Answer from the drawing. Dimensions are ordinates in mm from the lowest x, y and z of the part. Coordinates: 2 decimals unless noted, no trailing zeros. Write each loop counter-clockwise with the first axis right and the second up, starting at its lowest first coordinate (ties: lowest second). Pieces come first, ordered by that corner, then holes.
(1) For a pull along Y with two mould halves and no side action, classify the marked faces 1, 2 and 3 as +Y half, -Y half, draft (parallel to the pull), parting line (faces both ways), or undercut.
(2) Straight lines are drawn through the part: line 1 (X direction, y = 3, z = 36); line 2 (Y direction, x = 19, z = 32); line 3 (Y direction, x = 4, z = 6). For each, find the intervals that lie inside material, in ascending order.
(3) The part is cut by section C-C on z = 3.81. Give the number of separate pieces and of enclosed holes in the cut face, plus the area to 3 significant figures.
(4) The part is cut by section A-A on x = 19.05. Determine the outline of the cut face in (y, z), plus the area to 3 significant figures.
(5) Given P1, Ø4, axis at x = 28.575, z = 3.81, coming from the -Y side; P2, Ø4, axis at x = 9.525, z = 30.48, coming from the +Y side; P3, Ø7.5, axis at x = 19.05, y = 19.05, coming from the +Z side, each flat-ended and moving along its own axis, determine where each tip first touches the part or whether it passes through.
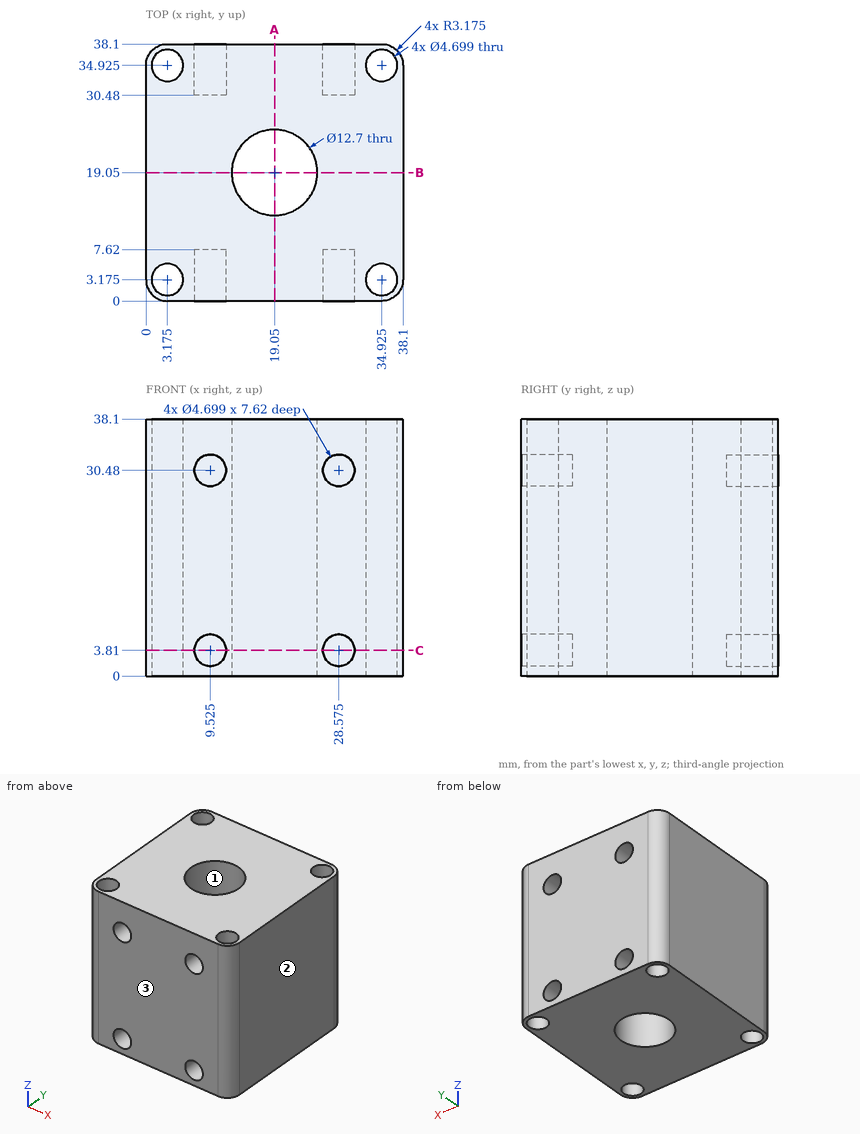
Model answer:
1. face 1: undercut
1. face 2: draft
1. face 3: -Y half
2. line 1: x = 0 to 0.83, 5.52 to 32.58, 37.27 to 38.1
2. line 2: y = 0 to 12.7, 25.4 to 38.1
2. line 3: y = 0 to 0.98, 5.37 to 32.73, 37.12 to 38.1
3. separate pieces: 1
3. enclosed holes: 5
3. area: 1,100 mm2
4. outline: (0, 0) - (12.7, 0) - (12.7, 38.1) - (0, 38.1) - close; (25.4, 0) - (38.1, 0) - (38.1, 38.1) - (25.4, 38.1) - close
4. area: 968 mm2
5. P1: stops at y = 7.62
5. P2: stops at y = 30.48
5. P3: passes through
